Read the model definition and answer for the solid it produces. Units are mm, in the model's axes. Face numbers are marked on the shaded views. Round coordinates to 2 decimals unless told otherwise and drop trailing zeros. Order: outer loops, then holes, each group sorted by start corner. A loop starts at its lowest first (then second) coordinate and runs counter-clockwise, first axis right, second up. Notation, with made-up numbers: (88, 85) -> (147, 85) arc R37 cw to (147, 122) -> close; hole circle Ø11 at (-17.5, 23). An arc over 180 degrees is marked (long way). One line per item, written item: value. Start each with the question number.
1. Flat-ended cylindrical pins translate along their axes: pin 1 Ø7.5 at (x, y) = (0, 0) entering from -Z; pin 2 Ø2 at (y, z) = (-7, 6.5) entering from +X; pin 3 Ø1 at (y, z) = (-6, 3.5) entering from +X. Find the tip coordinate at first contact, or state that the pin passes through.
2. Consider line 1 (X direction, y = -0.75, z = 11); line 2 (Y direction, x = 0, z = 4.25); line 3 (Y direction, x = -3.25, z = 1). Determine where each line is inside the solid, lowest interval first.
3. Section B-B (y = 0) is taken. State how many separate pieces and enclosed holes the cut face has, then the cut area to 3 significant figures.
4. Section A-A (x = 0) is taken. Give the vertices of the cut face in (y, z).
5. The mould has two halves that part along X. Classify the marked faces 1, 2 and 3: released by +X, released by -X, zero draft, split by the parting line, or undercut.
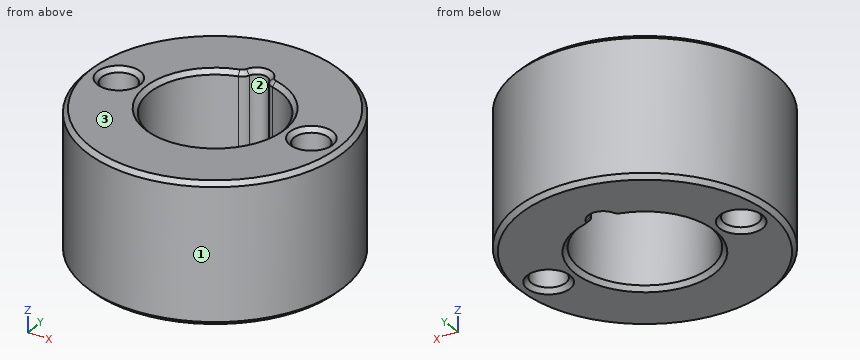
Autodesk Inventor part; units mm, degrees
ref_plane "YZ Plane" through (0, 0, 0) normal (1, 0, 0) x (0, 1, 0)
ref_plane "XZ Plane" through (0, 0, 0) normal (0, 1, 0) x (-1, 0, 0)
ref_plane "XY Plane" through (0, 0, 0) normal (0, 0, 1) x (1, 0, 0)
sketch "Эскиз1" plane through (0, 0, 0) normal (0, 0, 1) x (1, 0, 0)
  circle A0 centre (0, 0) radius 6.1
  circle A1 centre (0, 0) radius 12
  circle A2 centre (0, 0) radius 9 construction
  line L0 (-16.8, 0) -> (16.8, 0) construction
  circle A3 centre (-9, 0) radius 1.6
  circle A4 centre (9, 0) radius 1.6
  line L1 (0, -16.8) -> (0, 16.8) construction
  circle A5 centre (0, 6.1) radius 1
  point P0 (0.9966, 6.018)
  point P1 (-0.9966, 6.018)
  dimension "d0" = 12.2
  dimension "d1" = 24
  dimension "d2" = 18
  dimension "d3" = 3.2
  dimension "d4" = 3.2
  dimension "d10" = 2
extrude "Выдавливание1" add sketch "Эскиз1" along normal blind 13
fillet "Сопряжение1" radius 1 2 edges at (-0.9966, 6.018, 6.5) (0.9966, 6.018, 6.5)
chamfer "Фаска2" distance 0.4 angle 45 14 edges at (-1.1899, 6.105, 0) (1.1899, 6.105, 0) (0, -6.1, 0) (0, 7.1, 0) (-12, 0, 0) (7.4, 0, 0) (-10.6, 0, 0) (0, -6.1, 13) (-1.1899, 6.105, 13) (1.1899, 6.105, 13) (0, 7.1, 13) (-12, 0, 13) (-10.6, 0, 13) (7.4, 0, 13)
properties part number "Проставка шестерни"
Answer:
1. pin 1: through
1. pin 2: x = 10.39
1. pin 3: x = 10.67
2. line 1: -11.98 to -10.41, -7.59 to -6.05, 6.05 to 7.59, 10.41 to 11.98
2. line 2: -12 to -6.1, 7.1 to 12
2. line 3: -11.55 to -5.16, 5.16 to 11.55
3. separate pieces: 4
3. enclosed holes: 0
3. area: 68.9 mm^2
4. outline: (-12, 0.4) -> (-11.6, 0) -> (-6.5, 0) -> (-6.1, 0.4) -> (-6.1, 12.6) -> (-6.5, 13) -> (-11.6, 13) -> (-12, 12.6) -> close; (7.1, 0.4) -> (7.5, 0) -> (11.6, 0) -> (12, 0.4) -> (12, 12.6) -> (11.6, 13) -> (7.5, 13) -> (7.1, 12.6) -> close
5. face 1: split by the parting line
5. face 2: undercut
5. face 3: zero draft
